Drawing for the job (mm, zero at the part's lowest x, y, z). Coordinates: 2 decimals unless noted, no trailing zeros. Write each loop counter-clockwise with the first axis right and the second up, starting at its lowest first coordinate (ties: lowest second). Pieces come first, ordered by that corner, then holes.
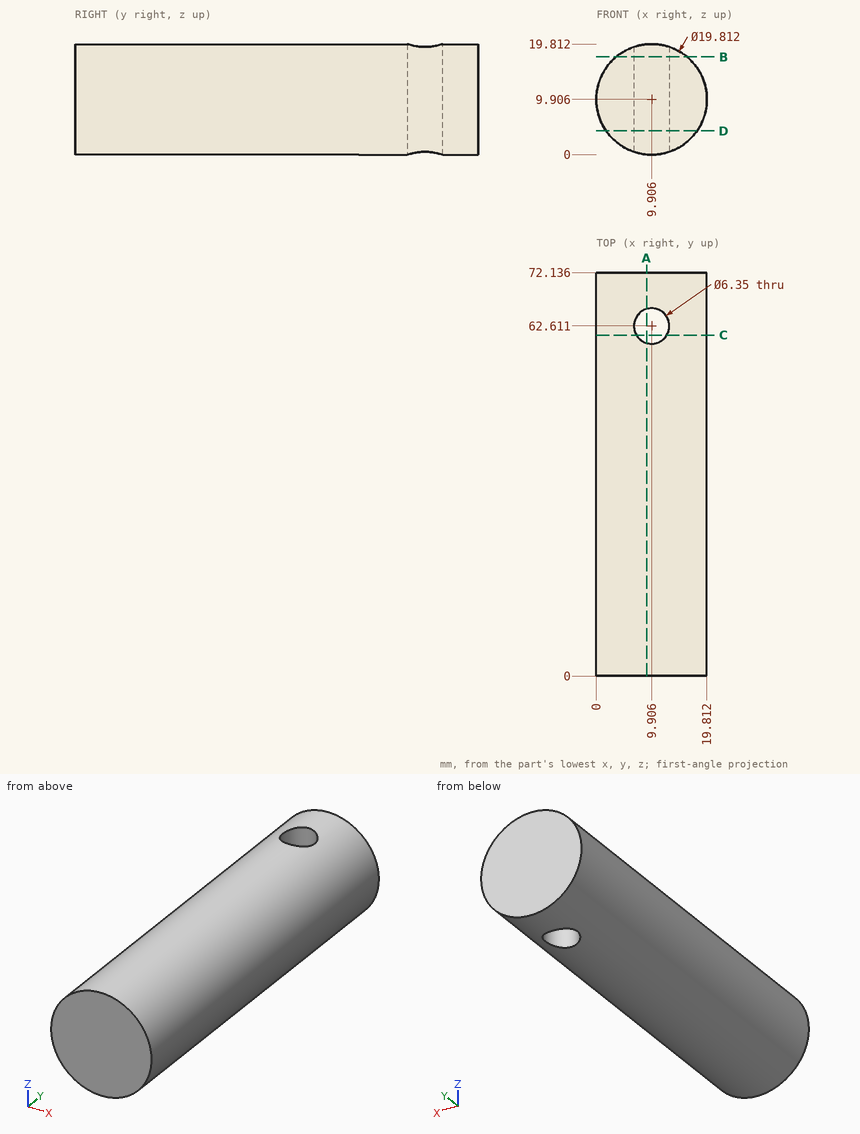
Item 1: Saw through at C-C, the plane y = 61. Write the cut outline in (x, z).
Item 2: Saw through at D-D, the plane z = 4.25. Write the cut outline in (x, y) (3 decimals), and give its area (3 significant figures).
Item 3: Saw through at B-B, the plane z = 17.5. Write the cut outline in (x, y) (3 decimals), and give its area (3 significant figures).
Item 4: Flat gauge pins, fed straight in: pin 1 Ø4 at (y, z) = (30.5, 16) entering from +X; pin 2 Ø3 at (x, y) = (5.5, 49) entering from -Z; pin 3 Ø2 at (x, y) = (14.5, 53) entering from +Z. Where does each tip first touch, or does it go through?
Item 5: Saw through at A-A, the plane x = 9. Write the cut outline in (y, z), and give its area (3 significant figures).
Item 6: Wall check: line 1 along Z through (x, y) = (9.75, 9); line 2 along X through (y, z) = (63, 2); line 3 along Y through (x, z) = (12.25, 2). Give the ranges that are in metal, low to high.
Working result:
1. outline: (7.17, 0.39) - (7.17, 19.43) arc R9.91 ccw to start; (12.64, 0.39) arc R9.91 ccw to (12.64, 19.43) - close
2. outline: (1.773, 0) - (18.039, 0) - (18.039, 72.136) - (1.773, 72.136) - close; hole circle Ø6.35 at (9.906, 62.611)
2. area: 1,140 mm2
3. outline: (3.545, 0) - (16.267, 0) - (16.267, 72.136) - (3.545, 72.136) - close; hole circle Ø6.35 at (9.906, 62.611)
3. area: 886 mm2
4. pin 1: stops at x = 18.93
4. pin 2: stops at z = 0.44
4. pin 3: stops at z = 19.14
5. outline: (0, 0.04) - (59.57, 0.04) - (59.57, 19.77) - (0, 19.77) - close; (65.65, 0.04) - (72.14, 0.04) - (72.14, 19.77) - (65.65, 19.77) - close
5. area: 1,300 mm2
6. line 1: z = 0 to 19.81
6. line 2: x = 3.94 to 6.75, 13.06 to 15.87
6. line 3: y = 0 to 60.47, 64.75 to 72.14
